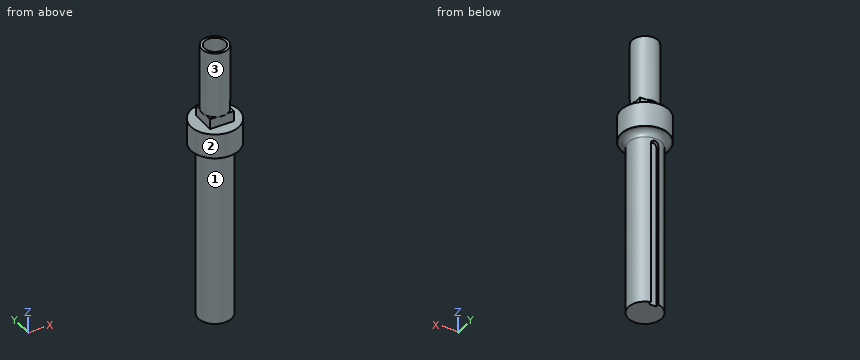
Autodesk Inventor part; units mm, degrees
ref_plane "Work Plane1" through (0, 12.7, 129.8575) normal (0, 0, 1) x (1, 0, 0)
ref_plane "YZ Plane" through (0, 0, 0) normal (1, 0, 0) x (0, 1, 0)
ref_plane "XZ Plane" through (0, 0, 0) normal (0, 1, 0) x (-1, 0, 0)
sketch "Sketch1" plane through (0, 0, 0) normal (0, 0, 1) x (1, 0, 0)
  circle A0 centre (0, 0) radius 12.7
  dimension "d0" = 25.4
extrude "Extrusion1" add sketch "Sketch1" along normal blind 155.575
sketch "Sketch2" plane through (0, 0, 155.575) normal (0, 0, 1) x (1, 0, 0)
  circle A0 centre (0, 0) radius 12.7
  line L0 (-8.9803, 8.9803) -> (8.9803, 8.9803)
  line L1 (8.9803, 8.9803) -> (8.9803, -8.9803)
  line L2 (8.9803, -8.9803) -> (-8.9803, -8.9803)
  line L3 (-8.9803, -8.9803) -> (-8.9803, 8.9803)
  line L4 (-8.9803, 8.9803) -> (8.9803, -8.9803) construction
  line L5 (8.9803, 8.9803) -> (-8.9803, -8.9803) construction
extrude "Extrusion2" add sketch "Sketch2" along normal blind 7.9375 contours L1 L2 L3 L0
sketch "Sketch3" plane through (0, 0, 163.5125) normal (0, 0, 1) x (1, 0, 0)
  circle A0 centre (0, 0) radius 9.9695
  dimension "d5" = 19.939
extrude "Extrusion3" add sketch "Sketch3" along normal blind 50.8
sketch "Sketch4" plane through (0, 0, 214.3125) normal (0, 0, 1) x (1, 0, 0)
  circle A0 centre (0, 0) radius 7.9375
  dimension "d8" = 15.875
extrude "Extrusion4" cut sketch "Sketch4" against normal up to surface (50.8 mm away)
sketch "Sketch5" plane through (0, 0, 0) normal (0, 0, -1) x (-1, 0, 0)
  line L0 (2.8575, 15.5575) -> (-2.8575, 15.5575)
  line L1 (-2.8575, 15.5575) -> (-2.8575, 9.8425)
  line L2 (-2.8575, 9.8425) -> (2.8575, 9.8425)
  line L3 (2.8575, 9.8425) -> (2.8575, 15.5575)
  arc A0 (8.9803, -8.9803) -> (8.9803, 8.9803) centre (0, 0) ccw
  line L4 (2.8575, 15.5575) -> (-2.8575, 9.8425) construction
  line L5 (-2.8575, 15.5575) -> (2.8575, 9.8425) construction
  point P0 (0, 12.7)
  point P1 (0, 12.7)
  dimension "d11" = 5.715
extrude "Extrusion5" cut sketch "Sketch5" against normal blind 129.8575
fillet "Fillet2" radius 2.8575 2 edges at (-2.8575, 11.1084, 129.8575) (2.8575, 11.1084, 129.8575)
sketch "Sketch6" plane through (0, 0, 155.575) normal (0, 0, 1) x (1, 0, 0)
  circle A0 centre (0, 0) radius 18.415
  dimension "d16" = 36.83
ref_plane "Work Plane1" through (0, 12.7, 129.8575) normal (0, 0, 1) x (1, 0, 0)
sketch "Sketch7" plane through (0, 12.7, 129.8575) normal (0, 0, 1) x (1, 0, 0)
  circle A0 centre (0, -12.7) radius 7.9375
  circle A1 centre (0, -12.7) radius 14.097
extrude "Extrusion6" add sketch "Sketch6" against normal blind 19.05
fillet "Fillet3" radius 4.7625 1 edges at (-12.7, 0, 136.525)
properties part number "Adam's Motor Shaft Rev2" material "Steel, Alloy"
Design review of the part built by this model. Coordinates are the model's own, in mm. Face numbers are marked on the shaded views. A direction names the side the tool comes from. Coordinates: 2 decimals unless noted, no trailing zeros. Order: outer loops, then holes, each group sorted by start corner. A loop starts at its lowest first (then second) coordinate and runs counter-clockwise, first axis right, second up.
Item 1: Take a section at D-D, the plane z = 110.5. Write out the cut boundary in (x, y), then the cut area to 3 significant figures.
Item 2: For line 1 (Y direction, x = 0, z = 204.5); line 2 (Z direction, x = -5, y = -6); line 3 (Z direction, x = -15, y = -8.5) (3 decimals), list the stretches that pass through material, from the lowest coordinate up.
Item 3: Take a section at B-B, the plane z = 185.5. Write out the cut boundary in (x, y) (1 decimal), then the cut area to 3 significant figures.
Item 4: Take a section at C-C, the plane z = 161. Write out the cut boundary in (x, y).
Item 5: For the marked faces 1, 2 and 3, list the 3-axis set-ups (+Z, -Z, +X, -X, +Y, -Y) from which the entire face can be reached by the end or side of a thin tool; tool diameter is ignored.
Item 6: For pin 1 Ø3 at (x, z) = (-1.5, 49.5) entering from +Y; pin 2 Ø2.5 at (y, z) = (-3, 160) entering from -X; pin 3 Ø8 at (x, z) = (14.5, 174) entering from +Y; pin 4 Ø8.5 at (x, z) = (1.5, 159.5) entering from -Y (3 decimals), all flat-tipped, find the tip position at first contact; note any pin that passes through.
Item 7: Take a section at A-A, the plane y = 0. Write out the cut boundary in (x, z) (1 decimal).
The answers:
1. outline: (-2.86, 9.84) - (-2.86, 12.37) arc R12.7 ccw (long way) to (2.86, 12.37) - (2.86, 9.84) - close
1. area: 491 mm2
2. line 1: y = -9.97 to -7.94, 7.94 to 9.97
2. line 2: z = 0 to 163.51
2. line 3: z = 136.52 to 155.575
3. outline: circle Ø19.9 at (0, 0); hole circle Ø15.9 at (0, 0)
3. area: 114 mm2
4. outline: (-8.98, -8.98) - (8.98, -8.98) - (8.98, 8.98) - (-8.98, 8.98) - close
5. face 1: -Z
5. face 2: +Z, -Z
5. face 3: +Z
6. pin 1: stops at y = 12.37
6. pin 2: stops at x = -8.98
6. pin 3: passes through
6. pin 4: stops at y = -18.415
7. outline: (-18.4, 136.5) - (-17.5, 136.5) arc R4.8 cw to (-12.7, 131.8) - (-12.7, 0) - (12.7, 0) - (12.7, 131.8) arc R4.8 cw to (17.5, 136.5) - (18.4, 136.5) - (18.4, 155.6) - (9, 155.6) - (9, 163.5) - (10, 163.5) - (10, 214.3) - (7.9, 214.3) - (7.9, 163.5) - (-7.9, 163.5) - (-7.9, 214.3) - (-10, 214.3) - (-10, 163.5) - (-9, 163.5) - (-9, 155.6) - (-18.4, 155.6) - close
